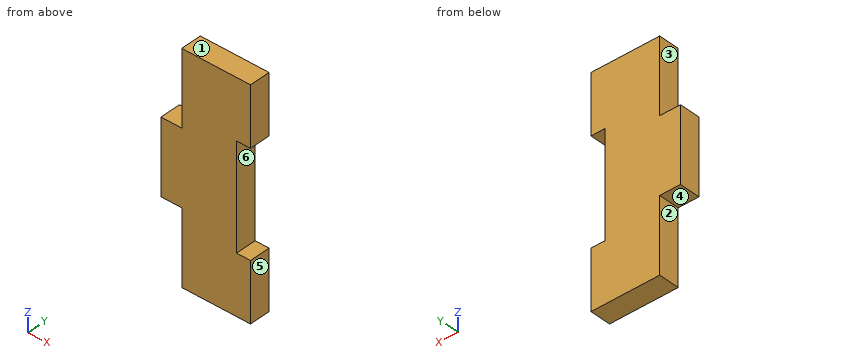
Autodesk Inventor part; units mm, degrees
ref_plane "YZ Plane" through (0, 0, 0) normal (1, 0, 0) x (0, 1, 0)
ref_plane "XZ Plane" through (0, 0, 0) normal (0, 1, 0) x (-1, 0, 0)
ref_plane "XY Plane" through (0, 0, 0) normal (0, 0, 1) x (1, 0, 0)
sketch "Esquisse1" plane through (0, 0, 0) normal (0, 1, 0) x (-1, 0, 0)
  line L0 (0, 0) -> (9.9, 0)
  line L1 (9.9, 0) -> (9.9, -32)
  line L2 (9.9, -32) -> (0, -32)
  line L3 (0, -32) -> (0, 0)
  line L4 (12.9, -21.3333) -> (9.9, -21.3333)
  line L5 (9.9, -21.3333) -> (9.9, -10.6667)
  line L6 (9.9, -10.6667) -> (12.9, -10.6667)
  line L7 (12.9, -10.6667) -> (12.9, -21.3333)
  point P0 (9.9, -16)
  dimension "d0" = 32
  dimension "d1" = 9.9
  dimension "d2" = 10.6667
  dimension "d3" = 3
extrude "Extrusion1" add sketch "Esquisse1" along normal blind 3
sketch "Esquisse2" plane through (0, 3, 0) normal (0, 1, 0) x (1, 0, 0)
  line L0 (-2, 8.5) -> (0, 8.5)
  line L1 (0, 8.5) -> (0, 23.5)
  line L2 (0, 23.5) -> (-2, 23.5)
  line L3 (-2, 23.5) -> (-2, 8.5)
  line L4 (-9.9, 21.3333) -> (-12.9, 21.3333)
  line L5 (-12.9, 21.3333) -> (-12.9, 10.6667)
  line L6 (-12.9, 10.6667) -> (-9.9, 10.6667)
  line L7 (-9.9, 10.6667) -> (-9.9, 0)
  line L8 (-9.9, 0) -> (0, 0)
  line L9 (0, 0) -> (0, 32)
  line L10 (0, 32) -> (-9.9, 32)
  line L11 (-9.9, 32) -> (-9.9, 21.3333)
  point P0 (0, 16)
  dimension "d6" = 2
  dimension "d7" = 15
extrude "Extrusion2" cut sketch "Esquisse2" against normal through all contours L3 L2 L1 L0
equation "\"d2\" = 0.333333 * d0"
properties part number "bottom_renfort"
Could you check a few things on this model? Use its own coordinates, in mm. Face numbers are marked on the shaded views. A direction names the side the tool comes from. Round coordinates to 2 decimals unless told otherwise and drop trailing zeros. Write each loop counter-clockwise with the first axis right and the second up, starting at its lowest first coordinate (ties: lowest second). Pieces come first, ordered by that corner, then holes. Notation, with made-up numbers: (28, -33.5) - (57, -33.5) arc R21 cw to (57, -12.5) - close; hole circle Ø1 at (47.5, 88.5). An arc over 180 degrees is marked (long way). Put each result on its own line as item: value. Start each with the question number.
(1) I want a section at C-C, the plane x = -11.25. Please give me the cut outline in (y, z).
(2) I want a section at B-B, the plane y = 2.35. Please give me the cut outline in (x, z).
(3) For the marked faces 1, 2 and 3, which set-ups out of +Z, -Z, +X, -X, +Y, -Y let a thin tool reach every point of the face, with its end or its side?
(4) Will these pins go through, and if not, where does the flat tip stop? pin 1 (0.6 mm diameter, centred on x = -1, y = 2, fed in from +Z); pin 2 (1.5 mm diameter, centred on y = 2, z = -29, fed in from -X).
(5) I want a section at D-D, the plane z = -23. Please give me the cut outline in (x, y), plus the area to 3 significant figures.
(6) Thinking about a two-plate mould opening in Z: for the marked faces 4, 5 and 6, which applies, released by +Z, released by -Z, zero draft, split by the parting line, or undercut?
(7) I want a section at A-A, the plane x = -1.5. Please give me the cut outline in (y, z), plus the area to 3 significant figures.
(8) I need wall thicknesses on probe 1 along Z at (x, y) = (-1.75, 2.3); probe 2 along X at (y, z) = (1.5, -3); probe 3 along X at (y, z) = (1.3, -12.5). Which ranges of each line are inside material? Lowest first, please.
Here are the results:
1. outline: (0, -21.33) - (3, -21.33) - (3, -10.67) - (0, -10.67) - close
2. outline: (-12.9, -21.33) - (-9.9, -21.33) - (-9.9, -32) - (0, -32) - (0, -23.5) - (-2, -23.5) - (-2, -8.5) - (0, -8.5) - (0, 0) - (-9.9, 0) - (-9.9, -10.67) - (-12.9, -10.67) - close
3. face 1: +Z, +X, -X, +Y, -Y
3. face 2: -Z, -X, +Y, -Y
3. face 3: +Z, -X, +Y, -Y
4. pin 1: stops at z = 0
4. pin 2: stops at x = -9.9
5. outline: (-9.9, 0) - (-2, 0) - (-2, 3) - (-9.9, 3) - close
5. area: 23.7 mm^2
6. face 4: released by -Z
6. face 5: zero draft
6. face 6: undercut
7. outline: (0, -32) - (3, -32) - (3, -23.5) - (0, -23.5) - close; (0, -8.5) - (3, -8.5) - (3, 0) - (0, 0) - close
7. area: 51.0 mm^2
8. probe 1: z = -32 to -23.5, -8.5 to 0
8. probe 2: x = -9.9 to 0
8. probe 3: x = -12.9 to -2
